The listing builds one solid part. Answer for the finished solid, in the listing's coordinates (mm). Face numbers are marked on the shaded views. A direction names the side the tool comes from. Coordinates: 2 decimals unless noted, no trailing zeros. Loops run counter-clockwise (first coordinate to the right, second up) from the corner with the lowest first, then second, coordinate; pieces in that order, holes last. Notation, with made-up numbers: (15, -5) - (20, -5) arc R28 ccw to (20, 32) - close; hole circle Ø10 at (28, 72.5). An arc over 180 degrees is marked (long way). One line per question, with ' | ' between items.
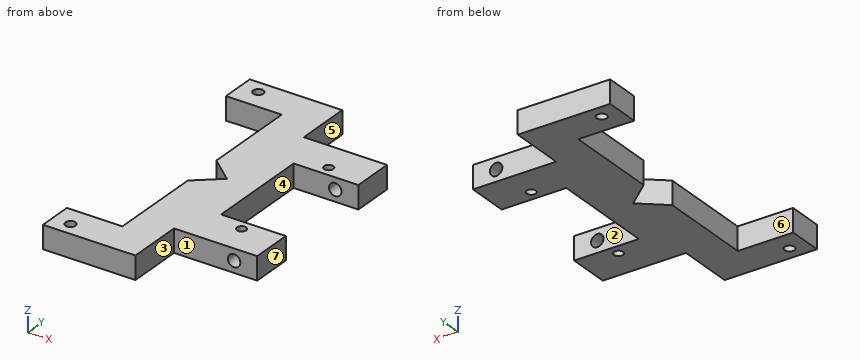
from build123d import *

# Parameters (mm, degrees)
F0_R     = 1
F1_DEPTH = 2.5
F3_DEPTH = 25
F6_DEPTH = 5
F7_R     = 1.1
F8_DEPTH = 5


with BuildPart() as f1:
    # F0 (on Top) → F1 (new body, symmetric)
    with BuildSketch(Plane.XY):
        Polygon((-7, -11.4), (-7, 11.4), (7, 11.4), (7, 20.4), (-11, 20.4), (-11, -20.4), (7, -20.4), (7, -11.4), align=None)
        with Locations((-1, -13.7)):
            Circle(F0_R, mode=Mode.SUBTRACT)
        with Locations((-1, 13.7)):
            Circle(F0_R, mode=Mode.SUBTRACT)
    extrude(amount=F1_DEPTH, both=True)

    # F2 (on Front) → F3 (cut, symmetric)
    with BuildSketch(Plane.XZ):
        with BuildLine():
            ThreePointArc((0.65, 0), (2, -1.35), (3.35, 0))
            ThreePointArc((3.35, 0), (2, 1.35), (0.65, 0))
        make_face()
    extrude(amount=F3_DEPTH, both=True, mode=Mode.SUBTRACT)

    # F5 (on offset) → F6 (join)
    with BuildSketch(Plane.XY.offset(2.5)):
        Polygon((-31, -25), (-31, -32.5), (-11, -32.5), (-11, 32.5), (-31, 32.5), (-31, 25), (-18.9318980411, 25), (-18.9598145062, 4.5039191309), (-13.6012034491, 0), (-18.9720636301, -4.4893051708), (-19, -25), align=None)
    extrude(amount=-F6_DEPTH)

    # F7 (on offset) → F8 (cut, through all)
    with BuildSketch(Plane.XY.offset(2.5)):
        with Locations((-27.1, 29.5)):
            Circle(F7_R)
        with Locations((-27.1, -29.5)):
            Circle(F7_R)
    extrude(amount=-F8_DEPTH, mode=Mode.SUBTRACT)


solid = f1.part
Item 1: Which of the six approach directions +Z, -Z, +X, -X, +Y, -Y give full straight-line access (tool end or side, diameter ignored) to the marked faces 4, 5, 6 and 7?
Taken from the geometry:
face 4: +Z, -Z, +X | face 5: +Z, -Z, +X, +Y | face 6: +Z, -Z, -X | face 7: +Z, -Z, +X, +Y, -Y
Item 2: The mould has two halves that part along Y. Classify the marked faces 1, 2 and 3: pulls with the +Y half, pulls with the -Y half, needs draft (parallel to the pull), parting line crosses it, or undercut.
Taken from the geometry:
face 1: pulls with the -Y half | face 2: undercut | face 3: needs draft
Item 3: Each of these flat-tipped pins is pushed along its axis until it touches: pin 1 Ø1.5 at (x, z) = (2, -1) entering from +Y; pin 2 Ø1.5 at (x, z) = (0.5, 0.5) entering from -Y; pin 3 Ø12 at (x, y) = (0, 1) entering from -Z; pin 4 Ø1.5 at (y, z) = (0.5, -0.5) entering from +X. Where does it stop, or does it pass through?
Taken from the geometry:
pin 1: stops at y = 20.4 | pin 2: stops at y = -20.4 | pin 3: passes through | pin 4: stops at x = -7
Item 4: Find section D-D, the plane x = -6. Write down the section's boundary in (y, z).
Taken from the geometry:
outline: (-20.4, -2.5) - (-11.4, -2.5) - (-11.4, 2.5) - (-20.4, 2.5) - close; (11.4, -2.5) - (20.4, -2.5) - (20.4, 2.5) - (11.4, 2.5) - close
Item 5: Find section A-A, the plane x = 2. Write down the section's boundary in (y, z).
Taken from the geometry:
outline: (-20.4, -2.5) - (-11.4, -2.5) - (-11.4, -1.35) - (-20.4, -1.35) - close; (-20.4, 1.35) - (-11.4, 1.35) - (-11.4, 2.5) - (-20.4, 2.5) - close; (11.4, -2.5) - (20.4, -2.5) - (20.4, -1.35) - (11.4, -1.35) - close; (11.4, 1.35) - (20.4, 1.35) - (20.4, 2.5) - (11.4, 2.5) - close
Item 6: Find section B-B, the plane y = 29.5. Write down the section's boundary in (x, z).
Taken from the geometry:
outline: (-31, -2.5) - (-28.2, -2.5) - (-28.2, 2.5) - (-31, 2.5) - close; (-26, -2.5) - (-11, -2.5) - (-11, 2.5) - (-26, 2.5) - close
Item 7: Find section C-C, the plane y = -13.7. Write down the section's boundary in (x, z), plus the area to 3 significant figures.
Taken from the geometry:
outline: (-18.98, -2.5) - (-2, -2.5) - (-2, 2.5) - (-18.98, 2.5) - close; (0, -2.5) - (7, -2.5) - (7, 2.5) - (0, 2.5) - close; hole circle Ø2.7 at (2, 0) | area: 114 mm2
Item 8: Find the intervals of material crossed by line 1 (Y direction, x = -27, z = -0.2); line 2 (Y direction, x = -1, z = -0.7); line 3 (Y direction, x = -3, z = 1.55), in increasing order. Write a range as [from, to].
Taken from the geometry:
line 1: y = [-32.5, -30.6], [-28.4, -25], [25, 28.4], [30.6, 32.5] | line 2: y = [-20.4, -14.7], [-12.7, -11.4], [11.4, 12.7], [14.7, 20.4] | line 3: y = [-20.4, -11.4], [11.4, 20.4]
